The drawing under review shows one solid part. Ordinate dimensions are in mm from its lowest x, y, z. A direction names the side the tool comes from. Coordinates: 2 decimals unless noted, no trailing zeros. Loops run counter-clockwise (first coordinate to the right, second up) from the corner with the lowest first, then second, coordinate; pieces in that order, holes last. Notation, with made-up numbers: (21, 6) - (34, 6) arc R6 ccw to (34, 12) - close; hole circle Ø4 at (59, 89.25). An arc over 180 degrees is marked (long way). Answer as a JSON object with one key per item and string values. Group by question number.
Item 1: We need section D-D (y = 16). Give the boundary of the cut face in (x, z), then the cut area to 3 significant figures.
Item 2: To check wall thickness, follow line 1 (Y direction, x = 11, z = 3.5); line 2 (Y direction, x = 11, z = 1.75); line 3 (Z direction, x = 11.5, y = 2.75). State the ranges of each line that lie inside material, in increasing order.
Item 3: We need section B-B (y = 11). Give the boundary of the cut face in (x, z), then the cut area to 3 significant figures.
Item 4: Mouldability with a two-part tool opening along X and no side actions: class the marked faces 1, 2 and 3 as released by +X, released by -X, zero draft, split by the parting line, or undercut.
Item 5: We need section A-A (x = 11). Give the boundary of the cut face in (y, z).
Item 6: We need section C-C (z = 1.55). Give the boundary of the cut face in (x, y).
Item 7: Clearance check with flat-ended pins moving along their axes: pin 1 (1.5 mm diameter, centred on y = 7, z = 3, fed in from -X); pin 2 (1.8 mm diameter, centred on x = 11, y = 16, fed in from +Z). State where each tip first meets the part, or that it passes through.
Item 8: Tool access review of the marked faces 4 and 5: name each direction out of +Z, -Z, +X, -X, +Y, -Y from which nothing blocks a thin tool from reaching the whole face with its end or side.
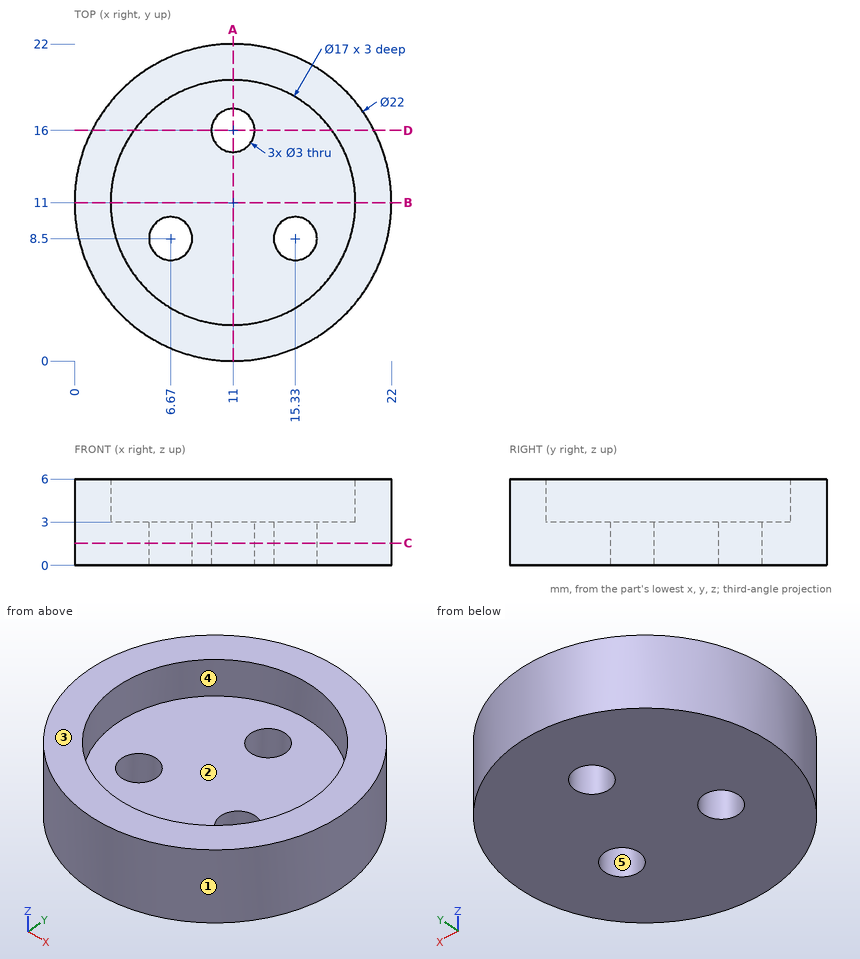
Check sheet entries:
{
 "1": {"outline": "(1.2, 0) - (9.5, 0) - (9.5, 3) - (4.13, 3) - (4.13, 6) - (1.2, 6) - close; (12.5, 0) - (20.8, 0) - (20.8, 6) - (17.87, 6) - (17.87, 3) - (12.5, 3) - close", "area": "67.3 mm2"},
 "2": {"line 1": "y = 0 to 2.5, 19.5 to 22", "line 2": "y = 0 to 14.5, 17.5 to 22", "line 3": "z = 0 to 3"},
 "3": {"outline": "(0, 0) - (22, 0) - (22, 6) - (19.5, 6) - (19.5, 3) - (2.5, 3) - (2.5, 6) - (0, 6) - close", "area": "81.0 mm2"},
 "4": {"face 1": "split by the parting line", "face 2": "undercut", "face 3": "zero draft"},
 "5": {"outline": "(0, 0) - (14.5, 0) - (14.5, 3) - (2.5, 3) - (2.5, 6) - (0, 6) - close; (17.5, 0) - (22, 0) - (22, 6) - (19.5, 6) - (19.5, 3) - (17.5, 3) - close"},
 "6": {"outline": "circle Ø22 at (11, 11); hole circle Ø3 at (6.67, 8.5); hole circle Ø3 at (11, 16); hole circle Ø3 at (15.33, 8.5)"},
 "7": {"pin 1": "stops at x = 0.49", "pin 2": "passes through"},
 "8": {"face 4": "+Z", "face 5": "+Z, -Z"}
}
